Check sheet for the modelled part. Datum: model origin and axes. Units: mm. Face numbers are marked on the shaded views. Give positions to 0.01 mm unless a question says otherwise; leave off trailing zeros. Order: outer loops, then holes, each group sorted by start corner. A loop starts at its lowest first (then second) coordinate and runs counter-clockwise, first axis right, second up. Notation, with made-up numbers: M -10,40 L 46,40 A20 ccw 46,75 Z; hole C 45.5,81 d6. An arc over 180 degrees is marked long. Return JSON: item names as keys, results as strings. Group by question number.
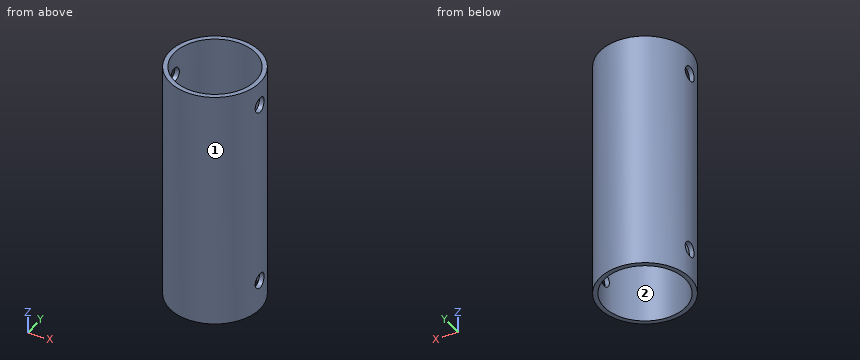
from build123d import *

# Parameters (mm, degrees)
SKETCH1_R           = 15
SKETCH1_R_2         = 13.5
BOSS_EXTRUDE1_DEPTH = 80
SKETCH2_R           = 2.5
CUT_EXTRUDE1_DEPTH  = 27


with BuildPart() as part:
    # Sketch1 → Boss-Extrude1 (new body)
    with BuildSketch(Plane.XY):
        Circle(SKETCH1_R)
        Circle(SKETCH1_R_2, mode=Mode.SUBTRACT)
    extrude(amount=BOSS_EXTRUDE1_DEPTH)

    # Sketch2 → Cut-Extrude1 (cut, symmetric)
    with BuildSketch(Plane(origin=(0, 0, 0), x_dir=(0, 0, -1), z_dir=(1, 0, 0))):
        with Locations((-10, 0)):
            Circle(SKETCH2_R)
        with Locations((-72, 0)):
            Circle(SKETCH2_R)
    extrude(amount=CUT_EXTRUDE1_DEPTH, both=True, mode=Mode.SUBTRACT)


solid = part.part
1) Material ranges on line 1 along X through (y, z) = (-0.5, 15); line 2 along Y through (x, z) = (0, 71); line 3 along Y through (x, z) = (11, 25), recorded low to high.
2) Sectioned sample at D-D on z = 31. Record the boundary of the cut face in (x, y).
3) Sectioned sample at A-A on y = 0. Record the boundary of the cut face in (x, z), then the cut area to 3 significant figures.
4) Sectioned sample at C-C on y = 12. Record the boundary of the cut face in (x, z).
5) Release check for a two-part mould opening along Y. For the marked faces 1 and 2 record: released by +Y, released by -Y, zero draft, split by the parting line, or undercut.
6) Depth check by flat-ended pin: P1, Ø12, axis at y = -12, z = 12.5, coming from the -X side; P2, Ø6, axis at y = 0, z = 72, coming from the -X side; P3, Ø1, axis at x = 9.5, z = 8.5, coming from the -Y side; P4, Ø4, axis at x = 8.5, z = 47.5, coming from the -Y side. Enter the tip coordinate at first touch or a pass-through.
7) Sectioned sample at B-B on x = 0. Record the boundary of the cut face in (y, z), then the cut area to 3 significant figures.
Reply:
{
 "1": {"line 1": "-14.99 to -13.49, 13.49 to 14.99", "line 2": "-15 to -13.5, 13.5 to 15", "line 3": "-10.2 to -7.83, 7.83 to 10.2"},
 "2": {"outline": "C 0,0 d30; hole C 0,0 d27"},
 "3": {"outline": "M -15,0 L -13.5,0 L -13.5,7.5 L -15,7.5 Z; M -15,12.5 L -13.5,12.5 L -13.5,69.5 L -15,69.5 Z; M -15,74.5 L -13.5,74.5 L -13.5,80 L -15,80 Z; M 13.5,0 L 15,0 L 15,7.5 L 13.5,7.5 Z; M 13.5,12.5 L 15,12.5 L 15,69.5 L 13.5,69.5 Z; M 13.5,74.5 L 15,74.5 L 15,80 L 13.5,80 Z", "area": "210 mm^2"},
 "4": {"outline": "M -9,0 L -6.18,0 L -6.18,80 L -9,80 Z; M 6.18,0 L 9,0 L 9,80 L 6.18,80 Z"},
 "5": {"face 1": "split by the parting line", "face 2": "undercut"},
 "6": {"P1": "x = -13.75", "P2": "x = -15", "P3": "y = -12", "P4": "y = -13.52"},
 "7": {"outline": "M -15,0 L -13.5,0 L -13.5,80 L -15,80 Z; M 13.5,0 L 15,0 L 15,80 L 13.5,80 Z", "area": "240 mm^2"}
}
